Source: CAD feature listing. Evaluate the final solid. Frame: model axes, mm. A direction names the side the tool comes from. Round coordinates to 2 decimals unless told otherwise and drop trailing zeros. Loops run counter-clockwise (first coordinate to the right, second up) from the corner with the lowest first, then second, coordinate; pieces in that order, holes last.
(1) Section D-D, the plane z = 0. Return the cut outline in (x, y).
(2) Section C-C, the plane y = -0.5. Return the cut outline in (x, z).
(3) Mould query, pull axis Z, two halves, no side actions, for faces 5 (the flat face through (10, 6.4, -24)), 6 (the flat face through (10, -9, 20)), 7 (the cylindrical face through (5.676, 5.414, 26.557)). Classes: pulls with the +Z half, pulls with the -Z half, needs draft (parallel to the pull), parting line crosses it, or undercut.
(4) Section B-B, the plane x = 5. Return the cut outline in (y, z), plus the area to 3 significant figures.
(5) Material intervals for probe 1 along Z at (x, y) = (7, -13.5); probe 2 along Y at (x, z) = (16.25, 21.5); probe 3 along Y at (x, z) = (6.75, 6.5), sorted ascending.
(6) First-contact query: pin 1 Ø6 at (x, z) = (13.5, 17) entering from +Y; pin 2 Ø4 at (x, z) = (15, 24.41) entering from +Y; pin 3 Ø1.8 at (x, z) = (10.5, 17.5) entering from +Y; pin 4 Ø6 at (x, y) = (14, -6) entering from -Z. Flat tips, straight axial feed; report the tip coordinate or a pass-through.
(7) Section A-A, the plane z = -8.5. Return the cut outline in (x, y), plus the area to 3 significant figures.
(8) Set-up query: faces 1 (the flat face through (2, 15, 14)), 2 (the flat face through (2, 13.1, -18)), 3 (the flat face through (10, 13.1, 17)), 4 (the flat face through (10, 4.4, 24)). Return all of +Z, -Z, +X, -X, +Y, -Y with unobstructed straight access to the full face (end or side cutting, diameter ignored); none if empty.
```python
from build123d import *

# Parameters (mm, degrees)
BOSS_EXTRUDE1_DEPTH = 20
SKETCH2_W           = 20
SKETCH2_H           = 40
CUT_EXTRUDE1_DEPTH  = 2.5
SKETCH3_W           = 20
SKETCH3_H           = 40
SKETCH3_R           = 3
CUT_EXTRUDE2_DEPTH  = 4
CUT_EXTRUDE3_DEPTH  = 4
SKETCH5_R           = 2.25
CUT_EXTRUDE4_DEPTH  = 2
CHAMFER1_SIZE       = 1.5


with BuildPart() as part:
    # Sketch1 → Boss-Extrude1 (new body)
    with BuildSketch(Plane(origin=(0, 0, 0), x_dir=(0, 0, -1), z_dir=(1, 0, 0))):
        Polygon((0, -23.6), (20, -23.6), (20, 4.4), (27, 4.4), (27, 6.4), (20, 6.4), (20, 12.4), (20, 23.6), (-20, 23.6), (-20, 12.4), (-20, 6.4), (-27, 6.4), (-27, 4.4), (-20, 4.4), (-20, -23.6), align=None)
    extrude(amount=BOSS_EXTRUDE1_DEPTH)

    # Sketch2 → Cut-Extrude1 (cut)
    with BuildSketch(Plane(origin=(0, 23.6, 0), x_dir=(1, 0, 0), z_dir=(0, 1, 0))):
        with Locations((10, 0)):
            Rectangle(SKETCH2_W, SKETCH2_H)
    extrude(amount=-CUT_EXTRUDE1_DEPTH, mode=Mode.SUBTRACT)

    # Sketch3 → Cut-Extrude2 (cut)
    with BuildSketch(Plane(origin=(0, 21.1, 0), x_dir=(1, 0, 0), z_dir=(0, 1, 0))):
        with Locations((10, 0)):
            Rectangle(SKETCH3_W, SKETCH3_H)
        with Locations(Location((10, 8.5, 0), (0, 0, 270))):
            Circle(SKETCH3_R, mode=Mode.SUBTRACT)
    extrude(amount=-CUT_EXTRUDE2_DEPTH, mode=Mode.SUBTRACT)

    # Sketch4 → Cut-Extrude3 (cut)
    with BuildSketch(Plane(origin=(0, 17.1, 0), x_dir=(1, 0, 0), z_dir=(0, 1, 0))):
        with BuildLine():
            Line((10.000000061, 20), (0, 20))
            Line((0, 20), (0, 14.178908346))
            ThreePointArc((0, 14.178908346), (4.214563395, 18.438748578), (10.000000061, 20))
        make_face()
        with BuildLine():
            Line((20, 20), (10.000000061, 20))
            ThreePointArc((10.000000061, 20), (15.785436657, 18.438748547), (20, 14.178908346))
            Line((20, 14.178908346), (20, 20))
        make_face()
        with BuildLine():
            Line((3.974014603, -14), (0, -14))
            Line((0, -14), (0, -20))
            Line((0, -20), (20, -20))
            Line((20, -20), (20, -14))
            Line((20, -14), (16.025985397, -14))
            ThreePointArc((16.025985397, -14), (10, -15.75), (3.974014603, -14))
        make_face()
    extrude(amount=-CUT_EXTRUDE3_DEPTH, mode=Mode.SUBTRACT)

    # Sketch5 → Cut-Extrude4 (cut)
    with BuildSketch(Plane(origin=(0, 6.4, 0), x_dir=(1, 0, 0), z_dir=(0, 1, 0))):
        with Locations(Location((5, -24.410545827, 0), (0, 0, 270))):
            Circle(SKETCH5_R)
        with Locations(Location((15, -24.410545827, 0), (0, 0, 270))):
            Circle(SKETCH5_R)
        with Locations(Location((15, 24.589454173, 0), (0, 0, 90))):
            Circle(SKETCH5_R)
        with Locations(Location((5, 24.589454173, 0), (0, 0, 90))):
            Circle(SKETCH5_R)
    extrude(amount=-CUT_EXTRUDE4_DEPTH, mode=Mode.SUBTRACT)

    # Chamfer1
    chamfer1_edges = [part.edges().sort_by_distance(p)[0] for p in [
        (0, -23.6, 0),
        (10, -23.6, 20),
        (10, -23.6, -20),
        (20, -23.6, 0),
    ]]
    chamfer(chamfer1_edges, length=CHAMFER1_SIZE)


solid = part.part
```
Output values:
1. outline: (0, -22.1) - (1.5, -23.6) - (18.5, -23.6) - (20, -22.1) - (20, 17.1) - (0, 17.1) - close
2. outline: (0, -20) - (20, -20) - (20, 20) - (0, 20) - close
3. face 5: needs draft
3. face 6: pulls with the +Z half
3. face 7: undercut
4. outline: (-23.6, -18.5) - (-22.1, -20) - (4.4, -20) - (4.4, -22.34) - (6.4, -22.34) - (6.4, -20) - (13.1, -20) - (13.1, -18.86) - (17.1, -18.86) - (17.1, 14.58) - (13.1, 14.58) - (13.1, 20) - (6.4, 20) - (6.4, 22.16) - (4.4, 22.16) - (4.4, 20) - (-22.1, 20) - (-23.6, 18.5) - close; (4.4, -27) - (6.4, -27) - (6.4, -26.84) - (4.4, -26.84) - close; (4.4, 26.66) - (6.4, 26.66) - (6.4, 27) - (4.4, 27) - close
4. area: 1,610 mm2
5. probe 1: z = -20 to 20
5. probe 2: y = 4.4 to 6.4
5. probe 3: y = -23.6 to 17.1
6. pin 1: stops at y = 17.1
6. pin 2: passes through
6. pin 3: stops at y = 13.1
6. pin 4: stops at z = -20
7. outline: (0, -22.1) - (1.5, -23.6) - (18.5, -23.6) - (20, -22.1) - (20, 17.1) - (13, 17.1) - (13, 21.1) - (7, 21.1) - (7, 17.1) - (0, 17.1) - close
7. area: 836 mm2
8. face 1: +Z, -X, +Y
8. face 2: -Z, -X, +Y
8. face 3: +Z, +Y
8. face 4: +Z, +X, -X, -Y
